Geometry: final body of the model. Coordinates: model frame, mm. Face numbers are marked on the shaded views. A direction names the side the tool comes from. Give positions to 0.01 mm unless a question says otherwise; leave off trailing zeros. Loops run counter-clockwise (first coordinate to the right, second up) from the corner with the lowest first, then second, coordinate; pieces in that order, holes last.
from build123d import *

# Parameters (mm, degrees)
F0_R     = 3.175
F0_R_2   = 4.75
F1_DEPTH = 20
F2_DEPTH = 30
F3_R     = 13
F4_DEPTH = 25


with BuildPart() as f1:
    # F0 (on Top) → F1 (new body)
    with BuildSketch(Plane.XY):
        with BuildLine():
            ThreePointArc((45.6904160883, -5.5314753587), (43.8303978971, -19.7324153288), (38.3758278236, -32.9753013065))
            Line((38.3758278236, -32.9753013065), (38.3758278236, -35.5302935839))
            Line((38.3758278236, -35.5302935839), (68.3758278236, -35.5302935839))
            Line((68.3758278236, -35.5302935839), (68.3758278236, 24.4697064161))
            Line((68.3758278236, 24.4697064161), (38.3758278236, 24.4697064161))
            Line((38.3758278236, 24.4697064161), (38.3758278236, 21.9123505891))
            ThreePointArc((38.3758278236, 21.9123505891), (43.8303978971, 8.6694646114), (45.6904160883, -5.5314753587))
        make_face()
        with Locations((61.3758278236, -5.5302935839)):
            Circle(F0_R, mode=Mode.SUBTRACT)
        with BuildLine():
            ThreePointArc((35.6904160883, -5.5314753587), (34.5069545017, -15.8000971879), (31.0186234261, -25.5302935839))
            Line((31.0186234261, -25.5302935839), (38.3758278236, -25.5302935839))
            Line((38.3758278236, -25.5302935839), (38.3758278236, -5.5302935839))
            Line((38.3758278236, -5.5302935839), (35.6904160728, -5.5302935839))
            ThreePointArc((35.6904160728, -5.5302935839), (35.6904160844, -5.5308844713), (35.6904160883, -5.5314753587))
        make_face()
        with BuildLine():
            ThreePointArc((-22.2183206005, 37.7662119119), (-25.8953821372, 36.5074722173), (-29.4505405381, 34.937104137))
            Line((-29.4505405381, 34.937104137), (-29.4505405381, -25.5302935839))
            Line((-29.4505405381, -25.5302935839), (-9.4505405381, -25.5302935839))
            Line((-9.4505405381, -25.5302935839), (31.0186234261, -25.5302935839))
            ThreePointArc((31.0186234261, -25.5302935839), (34.5069545017, -15.8000971879), (35.6904160883, -5.5314753587))
            ThreePointArc((35.6904160883, -5.5314753587), (35.6904160844, -5.5308844713), (35.6904160728, -5.5302935839))
            Line((35.6904160728, -5.5302935839), (20.5494594619, -5.5302935839))
            ThreePointArc((20.5494594619, -5.5302935839), (-0.6637439737, 3.2565029805), (-9.4505405381, 24.4697064161))
            Line((-9.4505405381, 24.4697064161), (-9.4505405381, 39.6094809703))
            ThreePointArc((-9.4505405381, 39.6094809703), (-12.8457783614, 39.4816149196), (-16.2217815185, 39.0987411975))
            ThreePointArc((-16.2217815185, 39.0987411975), (-18.7455341736, 36.2970945543), (-22.2183206005, 37.7662119119))
        make_face()
        with Locations((-19.4505405381, -15.5302935839)):
            Circle(F0_R_2, mode=Mode.SUBTRACT)
        Polygon((-1.4505405381, -10.5302935839), (8.5494594619, -10.5302935839), (-1.4505405381, -20.5302935839), align=None, mode=Mode.SUBTRACT)
        Polygon((25.5494594619, -20.5302935839), (15.5494594619, -20.5302935839), (25.5494594619, -10.5302935839), align=None, mode=Mode.SUBTRACT)
        Polygon((-24.4505405381, -1.5302935839), (-24.4505405381, 8.4697064161), (-14.4505405381, -1.5302935839), align=None, mode=Mode.SUBTRACT)
        Polygon((-14.4505405381, 25.4697064161), (-14.4505405381, 15.4697064161), (-24.4505405381, 25.4697064161), align=None, mode=Mode.SUBTRACT)
        with BuildLine():
            Line((-9.4505405381, 49.4697064161), (-13.3741952012, 49.4697064161))
            ThreePointArc((-13.3741952012, 49.4697064161), (-21.5481694996, 48.2660378849), (-29.4505405381, 45.8545641168))
            Line((-29.4505405381, 45.8545641168), (-29.4505405381, 34.937104137))
            ThreePointArc((-29.4505405381, 34.937104137), (-25.8953821372, 36.5074722173), (-22.2183206005, 37.7662119119))
            ThreePointArc((-22.2183206005, 37.7662119119), (-20.3357565561, 42.5968285118), (-16.2005405381, 39.4697064161))
            ThreePointArc((-16.2005405381, 39.4697064161), (-16.2058551286, 39.283919998), (-16.2217815185, 39.0987411975))
            ThreePointArc((-16.2217815185, 39.0987411975), (-12.8457783614, 39.4816149196), (-9.4505405381, 39.6094809703))
            Line((-9.4505405381, 39.6094809703), (-9.4505405381, 49.4697064161))
        make_face()
        with BuildLine():
            ThreePointArc((29.8809127675, 33.1151528142), (10.0506365578, 46.0459341182), (-13.3741952012, 49.4697064161))
            Line((-13.3741952012, 49.4697064161), (-9.4505405381, 49.4697064161))
            Line((-9.4505405381, 49.4697064161), (-9.4505405381, 39.6094809703))
            ThreePointArc((-9.4505405381, 39.6094809703), (22.4685181604, 26.3884188937), (35.6904160728, -5.5302935839))
            Line((35.6904160728, -5.5302935839), (38.3758278236, -5.5302935839))
            Line((38.3758278236, -5.5302935839), (38.3758278236, 21.9123505891))
            ThreePointArc((38.3758278236, 21.9123505891), (34.4868827374, 27.7856062501), (29.8809127675, 33.1151528142))
        make_face()
        with BuildLine():
            Line((-13.3741952012, 49.4697064161), (-29.4505405381, 49.4697064161))
            Line((-29.4505405381, 49.4697064161), (-29.4505405381, 45.8545641168))
            ThreePointArc((-29.4505405381, 45.8545641168), (-21.5481694996, 48.2660378849), (-13.3741952012, 49.4697064161))
        make_face()
        with BuildLine():
            Line((38.3758278236, 24.4697064161), (29.8809127675, 33.1151528142))
            ThreePointArc((29.8809127675, 33.1151528142), (34.4868827374, 27.7856062501), (38.3758278236, 21.9123505891))
            Line((38.3758278236, 21.9123505891), (38.3758278236, 24.4697064161))
        make_face()
    extrude(amount=F1_DEPTH)

    # F0 (on Top) → F2 (join)
    with BuildSketch(Plane.XY):
        with BuildLine():
            Line((38.3758278236, -25.5302935839), (38.3758278236, -32.9753013065))
            ThreePointArc((38.3758278236, -32.9753013065), (43.8303978971, -19.7324153288), (45.6904160883, -5.5314753587))
            ThreePointArc((45.6904160883, -5.5314753587), (43.8303978971, 8.6694646114), (38.3758278236, 21.9123505891))
            Line((38.3758278236, 21.9123505891), (38.3758278236, -5.5302935839))
            Line((38.3758278236, -5.5302935839), (38.3758278236, -25.5302935839))
        make_face()
        with BuildLine():
            ThreePointArc((45.6904160883, -5.5314753587), (43.8303978971, -19.7324153288), (38.3758278236, -32.9753013065))
            Line((38.3758278236, -32.9753013065), (38.3758278236, -35.5302935839))
            Line((38.3758278236, -35.5302935839), (68.3758278236, -35.5302935839))
            Line((68.3758278236, -35.5302935839), (68.3758278236, 24.4697064161))
            Line((68.3758278236, 24.4697064161), (38.3758278236, 24.4697064161))
            Line((38.3758278236, 24.4697064161), (38.3758278236, 21.9123505891))
            ThreePointArc((38.3758278236, 21.9123505891), (43.8303978971, 8.6694646114), (45.6904160883, -5.5314753587))
        make_face()
        with Locations((61.3758278236, -5.5302935839)):
            Circle(F0_R, mode=Mode.SUBTRACT)
    extrude(amount=F2_DEPTH)

    # F3 (on face) → F4 (cut)
    with BuildSketch(Plane.YZ.offset(68.3758278236)):
        with Locations((-5.5302935839, 15)):
            Circle(F3_R)
    extrude(amount=-F4_DEPTH, mode=Mode.SUBTRACT)


solid = f1.part
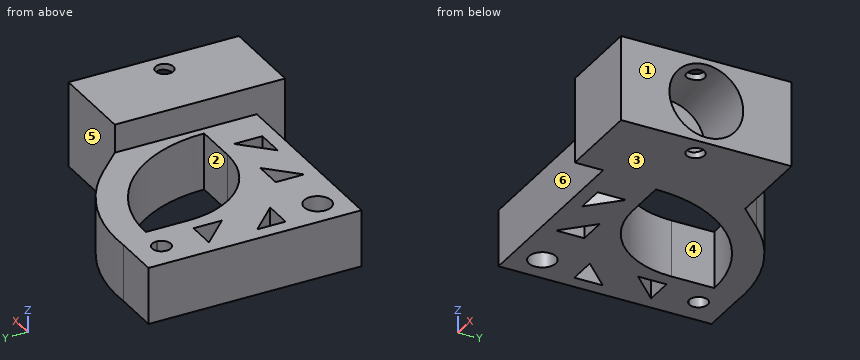
Item 1: Section query B-B on x = 46.5. Return loops of the section in (y, z).
Values follow:
outline: (-35.53, 0) - (24.47, 0) - (24.47, 30) - (-35.53, 30) - close; hole circle Ø26 at (-5.53, 15)
Item 2: Section query C-C on y = -12. Return loops of the section in (x, z).
Values follow:
outline: (-29.45, 0) - (-22.63, 0) - (-22.63, 20) - (-29.45, 20) - close; (-16.27, 0) - (-1.45, 0) - (-1.45, 20) - (-16.27, 20) - close; (7.08, 0) - (24.08, 0) - (24.08, 20) - (7.08, 20) - close; (25.55, 0) - (68.38, 0) - (68.38, 3.72) - (43.38, 3.72) - (43.38, 26.28) - (68.38, 26.28) - (68.38, 30) - (38.38, 30) - (38.38, 20) - (25.55, 20) - close
Item 3: Section query A-A on y = 32. Return loops of the section in (x, z).
Values follow:
outline: (-29.45, 0) - (-9.45, 0) - (-9.45, 20) - (-29.45, 20) - close; (15.63, 0) - (30.98, 0) - (30.98, 20) - (15.63, 20) - close
Item 4: Ray query, probe 1 along X at (y, z) = (1.5, 5); probe 2 along X at (y, z) = (0, 10); probe 3 along Y at (x, z) = (7.5, 5.5). Return the intervals inside material, ascending.
Values follow:
probe 1: x = -29.45 to -24.45, -17.48 to 1.25, 35.14 to 43.38
probe 2: x = -29.45 to -24.45, -15.98 to 3.19, 35.35 to 43.38
probe 3: y = -25.53 to -11.58, -10.53 to -2.54, 36.31 to 46.94
Item 5: Section query D-D on z = 15. Give the number of separate pieces and of enclosed holes in the cut face, plus the area to 3 significant figures.
Values follow:
separate pieces: 1
enclosed holes: 7
area: 4,150 mm2
Item 6: Pin query (flat end, axial travel): pin 1 (8 mm diameter, centred on y = 2.5, z = 13, fed in from +X); pin 2 (11 mm diameter, centred on x = -17, z = 12.5, fed in from +Y); pin 3 (16 mm diameter, centred on x = -2.5, z = 10.5, fed in from -Y). Return the tip coordinate at first contact, or that it passes through.
Values follow:
pin 1: stops at x = 43.38
pin 2: stops at y = 49.57
pin 3: stops at y = -25.53
Item 7: Draft query along X for the marked faces 1, 2 and 3. Return one class per face: +X half, -X half, draft (parallel to the pull), parting line (faces both ways), or undercut.
Values follow:
face 1: +X half
face 2: undercut
face 3: draft
Item 8: Set-up query: the marked faces 4, 5 and 6. Return all of +Z, -Z, +X, -X, +Y, -Y with unobstructed straight access to the full face (end or side cutting, diameter ignored); none if empty.
Values follow:
face 4: +Z, -Z
face 5: +Z, -Z, +X, +Y
face 6: +Z, -Z, -X, -Y
